Build history of the part. All positions in model axes, mm. A direction names the side the tool comes from. Round coordinates to 2 decimals unless told otherwise and drop trailing zeros. Write each loop counter-clockwise with the first axis right and the second up, starting at its lowest first coordinate (ties: lowest second). Pieces come first, ordered by that corner, then holes. Notation, with made-up numbers: (56, -18) - (65, -18) arc R11 ccw to (65, -4) - close; hole circle Ø8 at (33, 0.25). An arc over 180 degrees is marked (long way). Write each question's results on one line, items separated by ' | '.
Solid Edge part; units mm, degrees
sketch "Sketch1" plane through (0, 0, 0) normal (0, -1, 0) x (1, 0, 0)
  circle A0 centre (-6.3238, 0) radius 2.2
  line L0 (-31.7238, 7.2) -> (-0.3238, 7.2)
  line L1 (-0.3238, 7.2) -> (-0.3238, -7.2)
  line L2 (-0.3238, -7.2) -> (-31.7238, -7.2)
  line L3 (-31.7238, -7.2) -> (-31.7238, 7.2)
  circle A1 centre (-25.7238, 0) radius 2.2
  dimension "D1" = 25.7238
  dimension "D2" = 25.7238
  dimension "D3" = 6.3238
extrude "Protrusion1" add sketch "Sketch1" along normal blind 8
sketch "Sketch2" plane through (-14.9238, -8, 0) normal (0, -1, 0) x (1, 0, 0)
  line L0 (-14.4373, -2.1) -> (-14.4373, 2.1)
  line L1 (-14.4373, 2.1) -> (-10.8, 4.2)
  line L2 (-10.8, 4.2) -> (-7.1627, 2.1)
  line L3 (-7.1627, 2.1) -> (-7.1627, -2.1)
  line L4 (-7.1627, -2.1) -> (-10.8, -4.2)
  line L5 (-10.8, -4.2) -> (-14.4373, -2.1)
extrude "ExtrudedCutout_1" cut sketch "Sketch2" against normal blind 4
mirror "Mirror1" about plane through (-16.0238, -4, 0) normal (-1, 0, 0) of "ExtrudedCutout_1"
(1) Drill centre lines: probe 1 along X at (y, z) = (-1.15, 0); probe 2 along X at (y, z) = (-6.5, -1.5); probe 3 along Z at (x, y) = (-26.5, -2.5). Where is each one in solid material? Low to high. Write a range as [from, to].
Worked answers:
probe 1: x = [-31.72, -27.92], [-23.52, -8.52], [-4.12, -0.32] | probe 2: x = [-31.72, -29.36], [-22.09, -9.96], [-2.69, -0.32] | probe 3: z = [-7.2, -2.06], [2.06, 7.2]
(2) Slice it at D-D, the plane z = 2.5. Write the cut outline in (x, y).
Worked answers:
outline: (-31.72, -8) - (-28.67, -8) - (-28.67, -4) - (-22.78, -4) - (-22.78, -8) - (-9.27, -8) - (-9.27, -4) - (-3.38, -4) - (-3.38, -8) - (-0.32, -8) - (-0.32, 0) - (-31.72, 0) - close
(3) Tool access for faces 1 (the flat face through (-16, -8, 0)), 2 (the flat face through (-23.931, -6.028, 3.165)): list every direction of +Z, -Z, +X, -X, +Y, -Y with a clear straight run to the whole face (end or side of a thin tool).
Worked answers:
face 1: +Z, -Z, +X, -X, -Y | face 2: -Y
(4) Slice it at C-C, the plane x = -5. Write the cut outline in (y, z).
Worked answers:
outline: (-8, -7.2) - (0, -7.2) - (0, -1.76) - (-4, -1.76) - (-4, -3.44) - (-8, -3.44) - close; (-8, 3.44) - (-4, 3.44) - (-4, 1.76) - (0, 1.76) - (0, 7.2) - (-8, 7.2) - close
(5) Flat gauge pins, fed straight in: pin 1 Ø1 at (x, z) = (-4, -0.5) entering from +Y; pin 2 Ø2 at (x, z) = (-24.5, 0.5) entering from -Y. Where does each tip first touch, or does it go through?
Worked answers:
pin 1: stops at y = 0 | pin 2: stops at y = -4
(6) Two-plate mould, pull along Z, no slides. Class faces 3 (the flat face through (-16, 0, 0)), 4 (the flat face through (-29.361, -6, 0)), 5 (the cylindrical face through (-4.225, -1.972, -0.661)), 6 (the flat face through (-16, -4, 7.2)): released by +Z, released by -Z, zero draft, split by the parting line, or undercut.
Worked answers:
face 3: zero draft | face 4: undercut | face 5: undercut | face 6: released by +Z
(7) Slice it at B-B, the plane y = -1.5. Write the cut outline in (x, z), and give its area (3 significant figures).
Worked answers:
outline: (-31.72, -7.2) - (-0.32, -7.2) - (-0.32, 7.2) - (-31.72, 7.2) - close; hole circle Ø4.4 at (-25.72, 0); hole circle Ø4.4 at (-6.32, 0) | area: 422 mm2
(8) Slice it at A-A, the plane z = 0. Write the cut outline in (x, y).
Worked answers:
outline: (-31.72, -8) - (-29.36, -8) - (-29.36, -4) - (-27.92, -4) - (-27.92, 0) - (-31.72, 0) - close; (-23.52, -4) - (-22.09, -4) - (-22.09, -8) - (-9.96, -8) - (-9.96, -4) - (-8.52, -4) - (-8.52, 0) - (-23.52, 0) - close; (-4.12, -4) - (-2.69, -4) - (-2.69, -8) - (-0.32, -8) - (-0.32, 0) - (-4.12, 0) - close
